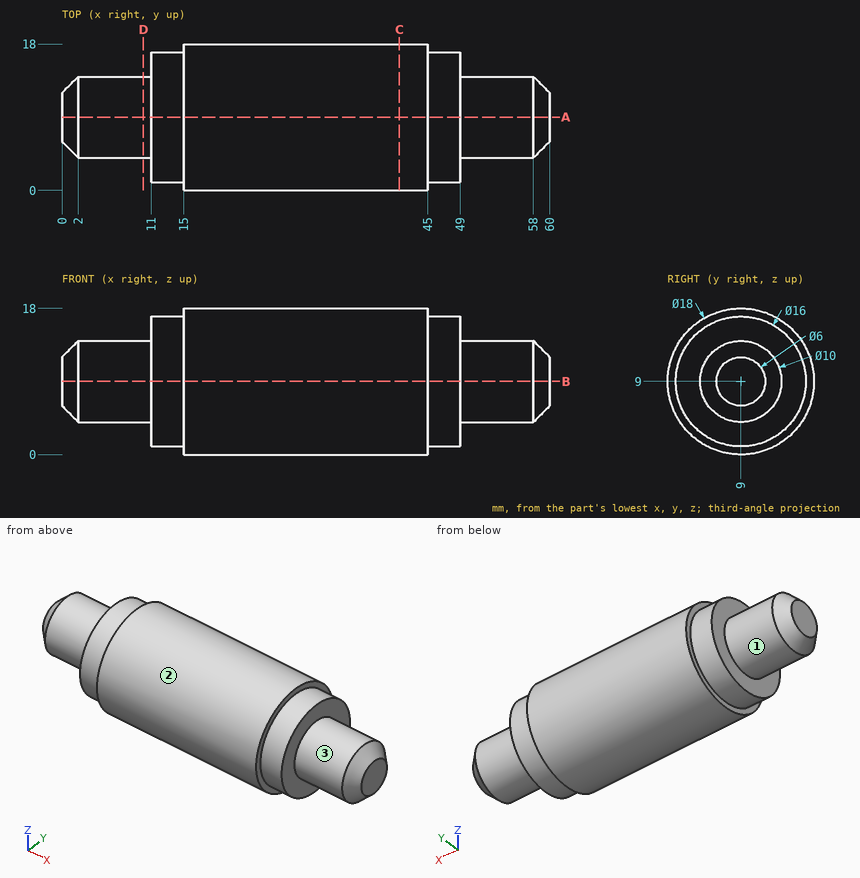
For this review, use the dimensioned drawing (mm, ordinates from the lowest corner) and the shaded views. A direction names the side the tool comes from. Give positions to 0.01 mm unless a question says otherwise; leave off trailing zeros. Loops run counter-clockwise (first coordinate to the right, second up) from the corner with the lowest first, then second, coordinate; pieces in that order, holes last. Notation, with made-up numbers: (72.5, 27) -> (92.5, 27) arc R20 ccw to (92.5, 43) -> close; hole circle Ø8 at (74.5, 81.5). An arc over 180 degrees is marked (long way). Use CSV: the item, a comma, the result in double quotes.
1. Consider section C-C, the plane x = 41.5. Write out the cut boundary in (y, z).
Result:
outline,"circle Ø18 at (9, 9)"
2. For P1, Ø2, axis at x = 44.5, z = 4, coming from the +Y side; P2, Ø4, axis at x = 49, y = 4.5, coming from the +Z side; P3, Ø5, axis at x = 24.5, z = 5.5, coming from the -Y side, all flat-tipped, find the tip position at first contact; note any pin that passes through.
Result:
P1,"stops at y = 17.06"
P2,"stops at z = 16.6"
P3,"stops at y = 0.06"
3. To check wall thickness, follow probe 1 along X at (y, z) = (3, 15); probe 2 along X at (y, z) = (2.5, 8.75); probe 3 along Z at (x, y) = (32.5, 9). State the ranges of each line that lie inside material, in increasing order. Write a range as from..to.
Result:
probe 1,"x = 15..45"
probe 2,"x = 11..49"
probe 3,"z = 0..18"
4. Machinability: for the marked faces 1, 2 and 3, which of the approach directions +Z, -Z, +X, -X, +Y, -Y give a long, thin tool a straight path to every point of the face, cutting with its end or side? Answer none if there is none.
Result:
face 1,"-X"
face 2,"+X, -X"
face 3,"+X"
5. Consider section D-D, the plane x = 10. Write out the cut boundary in (y, z), then the cut area to 3 significant figures.
Result:
outline,"circle Ø10 at (9, 9)"
area,"78.5 mm²"
6. Consider section A-A, the plane y = 9. Write out the cut boundary in (x, z), then the cut area to 3 significant figures.
Result:
outline,"(0, 6) -> (2, 4) -> (11, 4) -> (11, 1) -> (15, 1) -> (15, 0) -> (45, 0) -> (45, 1) -> (49, 1) -> (49, 4) -> (58, 4) -> (60, 6) -> (60, 12) -> (58, 14) -> (49, 14) -> (49, 17) -> (45, 17) -> (45, 18) -> (15, 18) -> (15, 17) -> (11, 17) -> (11, 14) -> (2, 14) -> (0, 12) -> close"
area,"880 mm²"
